from build123d import *

# Parameters (mm, degrees)
SKETCH_1_W          = 105
SKETCH_1_H          = 128
EXTRUDE_1_DEPTH     = 43
SKETCH_2_W          = 99
SKETCH_2_H          = 122
CUT_EXTRUDE_1_DEPTH = 50
SKETCH_3_W          = 99
SKETCH_3_H          = 2
EXTRUDE_2_DEPTH     = 90
CUT_EXTRUDE_2_REACH = 92.671
SKETCH_4_W          = 84
SKETCH_4_H          = 70
SKETCH_5_W          = 99
SKETCH_5_H          = 3
EXTRUDE_3_DEPTH     = 3
SKETCH_6_W          = 15
SKETCH_6_H          = 8
CUT_EXTRUDE_3_DEPTH = 10
SKETCH_8_W          = 84
SKETCH_8_H          = 8.5
CUT_EXTRUDE_4_DEPTH = 2
EXTRUDE_4_REACH     = 129.863
SKETCH_9_W          = 2
SKETCH_9_H          = 122
SKETCH_10_W         = 87
SKETCH_10_H         = 110
CUT_EXTRUDE_5_DEPTH = 8
FILLET_10_R         = 10
FILLET_11_R         = 20
FILLET_12_R         = 20
FILLET_13_R         = 10
FILLET_14_R         = 20
FILLET_15_R         = 20
FILLET_16_R         = 20


with BuildPart() as part:
    # 草图1 → 凸台-拉伸1 (new body)
    with BuildSketch(Plane.XY):
        Rectangle(SKETCH_1_W, SKETCH_1_H)
    extrude(amount=EXTRUDE_1_DEPTH)

    # 草图2 → 切除-拉伸1 (cut)
    with BuildSketch(Plane.XY.offset(43)):
        Rectangle(SKETCH_2_W, SKETCH_2_H)
    extrude(amount=-CUT_EXTRUDE_1_DEPTH, mode=Mode.SUBTRACT)

    # 草图3 → 凸台-拉伸2 (add)
    with BuildSketch(Plane.XZ.offset(-61)):
        with Locations((0, 36)):
            Rectangle(SKETCH_3_W, SKETCH_3_H)
    extrude(amount=EXTRUDE_2_DEPTH)

    # 草图4 → 切除-拉伸2 (cut, up to next)
    with BuildSketch(Plane.XY.offset(37), mode=Mode.PRIVATE) as cut_extrude_2_sk1:
        with Locations((0, 17.5)):
            Rectangle(SKETCH_4_W, SKETCH_4_H)
    cut_extrude_2_tool1 = extrude(cut_extrude_2_sk1.sketch, amount=-CUT_EXTRUDE_2_REACH, mode=Mode.PRIVATE) & part.part
    add(cut_extrude_2_tool1.solids().sort_by_distance((0, 17.5, 37))[0], mode=Mode.SUBTRACT)

    # 草图5 → 凸台-拉伸3 (add)
    with BuildSketch(Plane.XY.offset(37)):
        with Locations((0, -27.5)):
            Rectangle(SKETCH_5_W, SKETCH_5_H)
    extrude(amount=EXTRUDE_3_DEPTH)

    # 草图6 → 切除-拉伸3 (cut)
    with BuildSketch(Plane(origin=(0, 64, 0), x_dir=(1, 0, 0), z_dir=(0, 1, 0))):
        with Locations((0, -24)):
            Rectangle(SKETCH_6_W, SKETCH_6_H)
    extrude(amount=-CUT_EXTRUDE_3_DEPTH, mode=Mode.SUBTRACT)

    # 草图8 → 切除-拉伸4 (cut)
    with BuildSketch(Plane.XY.offset(37)):
        with Locations((0, 56.75)):
            Rectangle(SKETCH_8_W, SKETCH_8_H)
    extrude(amount=-CUT_EXTRUDE_4_DEPTH, mode=Mode.SUBTRACT)

    # 草图9 → 凸台-拉伸4 (add, up to next)
    with BuildSketch(Plane.ZY.offset(-49.5), mode=Mode.PRIVATE) as extrude_4_sk1:
        with Locations((4, 0)):
            Rectangle(SKETCH_9_W, SKETCH_9_H)
    extrude_4_tool1 = extrude(extrude_4_sk1.sketch, amount=EXTRUDE_4_REACH, mode=Mode.PRIVATE) - part.part
    add(extrude_4_tool1.solids().sort_by_distance((49.5, 0, 4))[0])

    # 草图10 → 切除-拉伸5 (cut)
    with BuildSketch(Plane(origin=(0, 0, 3), x_dir=(-1, 0, 0), z_dir=(0, 0, -1))):
        Rectangle(SKETCH_10_W, SKETCH_10_H)
    extrude(amount=-CUT_EXTRUDE_5_DEPTH, mode=Mode.SUBTRACT)

    # 圆角10
    fillet_10_edges = [part.edges().sort_by_distance(p)[0] for p in [
        (-52.5, -64, 21.5),
    ]]
    fillet(fillet_10_edges, radius=FILLET_10_R)

    # 圆角11
    fillet_11_edges = [part.edges().sort_by_distance(p)[0] for p in [
        (-49.5, -61, 1.5),
    ]]
    fillet(fillet_11_edges, radius=FILLET_11_R)

    # 圆角12
    fillet_12_edges = [part.edges().sort_by_distance(p)[0] for p in [
        (49.5, -61, 1.5),
    ]]
    fillet(fillet_12_edges, radius=FILLET_12_R)

    # 圆角13
    fillet_13_edges = [part.edges().sort_by_distance(p)[0] for p in [
        (52.5, -64, 21.5),
    ]]
    fillet(fillet_13_edges, radius=FILLET_13_R)

    # 圆角14
    fillet_14_edges = [part.edges().sort_by_distance(p)[0] for p in [
        (-49.5, 61, 1.5),
        (49.5, 61, 1.5),
    ]]
    fillet(fillet_14_edges, radius=FILLET_14_R)

    # 圆角15
    fillet_15_edges = [part.edges().sort_by_distance(p)[0] for p in [
        (49.5, -61, 24),
    ]]
    fillet(fillet_15_edges, radius=FILLET_15_R)

    # 圆角16
    fillet_16_edges = [part.edges().sort_by_distance(p)[0] for p in [
        (-49.5, -61, 24),
    ]]
    fillet(fillet_16_edges, radius=FILLET_16_R)


solid = part.part
Build history of the part. All positions in model axes, mm. A direction names the side the tool comes from. Round coordinates to 2 decimals unless told otherwise and drop trailing zeros. Write each loop counter-clockwise with the first axis right and the second up, starting at its lowest first coordinate (ties: lowest second). Pieces come first, ordered by that corner, then holes. Notation, with made-up numbers: M 48,-10 L 75,-10 A13 cw 75,2 Z; hole C -8.75,-26 d2. An arc over 180 degrees is marked long. Answer as a JSON object with one key per item and string values. Group by question number.
(1) Flat gauge pins, fed straight in: pin 1 (0.9 mm diameter, centred on x = -8, y = -27, fed in from +Z); pin 2 (3.5 mm diameter, centred on x = 1, y = 62, fed in from -Z); pin 3 (10 mm diameter, centred on x = -37.5, y = 9.5, fed in from -Z). Where does each tip first touch, or does it go through?
(2) Cut at A-A (z = 12). Give the cut face in (x, y), and give its area (3 significant figures).
(3) Cut at C-C (y = 49.5). Give the cut face in (x, z).
(4) Which spindle directions (+Z, -Z, +X, -X, +Y, -Y) get a long thin tool onto all of the face, cutting with end or side? Do faces 1 (the flat face through (-1, -27, 40)), 2 (the flat face through (0, 63, 20)), 3 (the flat face through (-49.5, -1, 2)). Say none if no direction does.
(5) Drill centre lines: L1, parallel to Y at x = -27, z = 37.5; L2, parallel to X at y = 18, z = 9; L3, parallel to X at y = 47.5, z = 35.5. Where is each one in solid material? Low to high.
(6) Cut at B-B (x = 11.5). Give the cut face in (y, z).
(7) Mould opens along Y. For faces 4 (the flat face through (-49.5, 9, 24)), 5 (the cylindrical face through (49.49, -61.15, 21.8)), 6 (the flat face through (7.5, 63, 24)) say: pulls with the +Y half, pulls with the -Y half, needs draft (parallel to the pull), parting line crosses it, or undercut.
(8) Cut at D-D (z = 24.5). Give the cut face in (x, y).
Responses:
{
 "1": {"pin 1": "stops at z = 40", "pin 2": "stops at z = 0", "pin 3": "stops at z = 35"},
 "2": {"outline": "M -52.5,-54 A10 ccw -42.5,-64 L 42.5,-64 A10 ccw 52.5,-54 L 52.5,64 L -52.5,64 Z; hole M -49.5,-41 A20 ccw -29.5,-61 L 29.5,-61 A20 ccw 49.5,-41 L 49.5,61 L -49.5,61 Z", "area": "1,490 mm2"},
 "3": {"outline": "M -52.5,0 L -47.6,0 L -47.6,3 L -43.5,3 L -43.5,5 L -49.5,5 L -49.5,35 L -42,35 L -42,37 L -49.5,37 L -49.5,43 L -52.5,43 Z; M 42,35 L 49.5,35 L 49.5,5 L 43.5,5 L 43.5,3 L 47.6,3 L 47.6,0 L 52.5,0 L 52.5,43 L 49.5,43 L 49.5,37 L 42,37 Z"},
 "4": {"face 1": "+Z", "face 2": "+Y", "face 3": "-Z"},
 "5": {"L1": "y = -64 to -61, -29 to -26, 61 to 64", "L2": "x = -52.5 to -49.5, 49.5 to 52.5", "L3": "x = -52.5 to -42, 42 to 52.5"},
 "6": {"outline": "M -64,0 L -61,0 L -61,3 L -55,3 L -55,5 L -61,5 L -61,43 L -64,43 Z; M -29,35 L -17.5,35 L -17.5,37 L -26,37 L -26,40 L -29,40 Z; M 55,3 L 61,3 L 61,0 L 64,0 L 64,43 L 61,43 L 61,5 L 55,5 Z"},
 "7": {"face 4": "undercut", "face 5": "pulls with the -Y half", "face 6": "needs draft"},
 "8": {"outline": "M -52.5,-54 A10 ccw -42.5,-64 L 42.5,-64 A10 ccw 52.5,-54 L 52.5,64 L 7.5,64 L 7.5,61 L 49.5,61 L 49.5,-41 A20 cw 29.5,-61 L -29.5,-61 A20 cw -49.5,-41 L -49.5,61 L -7.5,61 L -7.5,64 L -52.5,64 Z"}
}
